from build123d import *

# Parameters (mm, degrees)
CROQUIS1_R              = 9.8
CROQUIS1_R_2            = 1.61
CROQUIS1_R_3            = 1.610199264
CROQUIS1_R_4            = 1.610298895
SALIENTE_EXTRUIR2_DEPTH = 2.5


with BuildPart() as part:
    # Croquis1 → Saliente-Extruir2 (new, symmetric)
    with BuildSketch(Plane(origin=(0, 0, 0), x_dir=(1, 0, 0), z_dir=(0, 1, 0))):
        Polygon((-20.192989013, 7.194690523), (-10.192989013, 7.194690523), (-10.192989013, 11.914690523), (10.237010987, 11.914690523), (10.237010987, 6.914690523), (20.237010987, 6.914690523), (20.237010987, -12.805309477), (-20.192989013, -12.805309477), align=None)
        with Locations(Location((0, -1.965309477, 0), (0, 0, 270))):
            Circle(CROQUIS1_R, mode=Mode.SUBTRACT)
        with Locations(Location((-12.339891833, 5.049690523, 0), (0, 0, 270))):
            Circle(CROQUIS1_R_2, mode=Mode.SUBTRACT)
        with Locations(Location((-12.339891833, -10.660508741, 0), (0, 0, 270))):
            Circle(CROQUIS1_R_3, mode=Mode.SUBTRACT)
        with Locations(Location((15.290108167, 5.049690523, 0), (0, 0, 270))):
            Circle(CROQUIS1_R_2, mode=Mode.SUBTRACT)
        with Locations(Location((15.290108167, -10.660608373, 0), (0, 0, 270))):
            Circle(CROQUIS1_R_4, mode=Mode.SUBTRACT)
        with Locations(Location((-7.653762012, 9.553535498, 0), (0, 0, 270))):
            Circle(CROQUIS1_R_4, mode=Mode.SUBTRACT)
        with Locations(Location((7.645768396, 9.553535498, 0), (0, 0, 270))):
            Circle(CROQUIS1_R_4, mode=Mode.SUBTRACT)
    extrude(amount=SALIENTE_EXTRUIR2_DEPTH, both=True)


solid = part.part
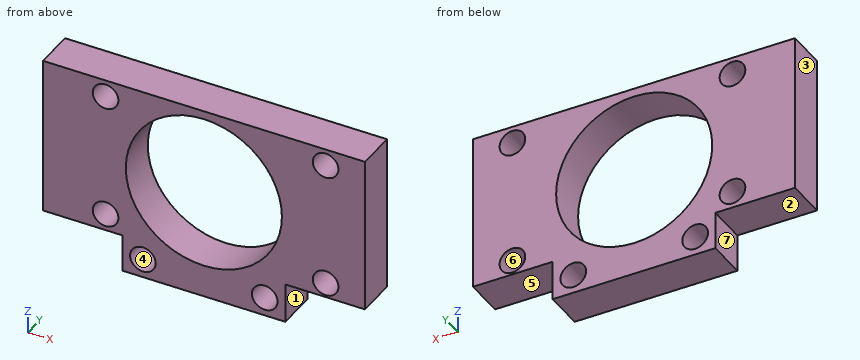
Input: part model. Units: mm. Frame: model coordinates. Face numbers are marked on the shaded views. A direction names the side the tool comes from. Round coordinates to 2 decimals unless told otherwise and drop trailing zeros. Loops run counter-clockwise (first coordinate to the right, second up) from the corner with the lowest first, then second, coordinate; pieces in that order, holes last. Notation, with made-up numbers: M -28.5,46 L -16.5,46 A12 ccw -16.5,64 Z; hole C 77.25,53.5 d9. An arc over 180 degrees is marked long. Answer as CSV lines item,"result". Start each with the question number.
(1) Draft query along X for the marked faces 4, 5, 6 and 7. Return one class per face: released by +X, released by -X, zero draft, split by the parting line, or undercut.
(2) Reachability of the marked faces 1, 2 and 3 from +Z, -Z, +X, -X, +Y, -Y: full face, straight path, thin tool, end or side. Return the list, or none.
(3) Line query: line 1 (X direction, y = -0.5, z = -6.5); line 2 (X direction, y = 1.2, z = 2); line 3 (Z direction, x = 9, y = 1.9). Output: solid intervals per line, ascending. Write a range as [from, to].
(4) Section D-D, the plane y = -1.95. Output: boundary loops of the cut face in (x, z).
(5) Section B-B, the plane z = 6.75. Output: boundary loops of the cut face in (x, y), plus the area to 3 significant figures.
(6) First-contact query: pin 1 (12 mm diameter, centred on x = 0, z = 1.97, fed in from -Y); pin 2 (1.5 mm diameter, centred on y = 1, z = -9.5, fed in from +X); pin 3 (1.5 mm diameter, centred on x = -14.5, y = -0.5, fed in from -Z). Flat tips, straight axial feed; report the tip coordinate or a pass-through.
(7) Section A-A, the plane x = 0. Output: boundary loops of the cut face in (y, z), plus the area to 3 significant figures.
(8) Section C-C, the plane x = -11.5. Output: boundary loops of the cut face in (y, z), plus the area to 3 significant figures.
Values found:
1,face 4,"undercut"
1,face 5,"zero draft"
1,face 6,"undercut"
1,face 7,"released by -X"
2,face 1,"-Z, +X, +Y, -Y"
2,face 2,"-Z, -X, +Y, -Y"
2,face 3,"+Z, -Z, -X, +Y, -Y"
3,line 1,"x = [-20.19, -13.04], [-11.64, -4.94], [4.94, 14.59], [15.99, 20.24]"
3,line 2,"x = [-20.19, -9.8], [9.8, 20.24]"
3,line 3,"z = [-11.91, -10.42], [-8.68, -1.91], [5.84, 12.81]"
4,outline,"M -20.19,-7.19 L -10.19,-7.19 L -10.19,-11.91 L 10.24,-11.91 L 10.24,-6.91 L 20.24,-6.91 L 20.24,12.81 L -20.19,12.81 Z; hole C -12.34,-5.05 d3.22; hole C -12.34,10.66 d3.22; hole C 0,1.97 d19.6; hole C -7.65,-9.55 d3.22; hole C 7.65,-9.55 d3.22; hole C 15.29,-5.05 d3.22; hole C 15.29,10.66 d3.22"
5,outline,"M -20.19,-2.5 L -8.55,-2.5 L -8.55,2.5 L -20.19,2.5 Z; M 8.55,-2.5 L 20.24,-2.5 L 20.24,2.5 L 8.55,2.5 Z"
5,area,"117 mm²"
6,pin 1,"passes through"
6,pin 2,"stops at x = 10.24"
6,pin 3,"stops at z = -7.19"
7,outline,"M -2.5,-11.91 L 2.5,-11.91 L 2.5,-7.83 L -2.5,-7.83 Z; M -2.5,11.77 L 2.5,11.77 L 2.5,12.81 L -2.5,12.81 Z"
7,area,"25.6 mm²"
8,outline,"M -2.5,-7.19 L 2.5,-7.19 L 2.5,-6.42 L -2.5,-6.42 Z; M -2.5,-3.68 L 2.5,-3.68 L 2.5,9.29 L -2.5,9.29 Z; M -2.5,12.03 L 2.5,12.03 L 2.5,12.81 L -2.5,12.81 Z"
8,area,"72.5 mm²"
